For this review, take the finished solid that the model builds, in its own axes (mm). A direction names the side the tool comes from. Give positions to 0.01 mm unless a question says otherwise; leave off trailing zeros. Order: outer loops, then holes, each group sorted by start corner. A loop starts at its lowest first (then second) coordinate and runs counter-clockwise, first axis right, second up. Notation, with made-up numbers: (45.25, 40.25) - (54.25, 40.25) arc R23 ccw to (54.25, 67.25) - close; hole circle Ø5 at (0, -5.75). An arc over 180 degrees is marked (long way). Use a Markdown table: item, result. Add a question column.
1) We need section C-C on z = -87.5. Write out the cut boundary in (x, y).
2) Wall thickness on L1, parallel to Z at x = -18, y = 3.75; L2, parallel to X at y = 2.5, z = -98.5; L3, parallel to X at y = 3.25, z = -45.5: over which ranges is each line inside the solid? List them lowest first.
3) Clearance check with flat-ended pins moving along their axes: P1, Ø3.5, axis at x = -18.01, z = -37.86, coming from the +Y side; P2, Ø2, axis at y = 2.5, z = -77, coming from the +X side. State where each tip first meets the part, or that it passes through.
4) Mouldability with a two-part tool opening along Z and no side actions: class faces 4 (the face through (-37, 3, -102.633)), 5 (the face through (28.728, 3, -68)), 6 (the face through (-37, 3, -32.783)), 7 (the face through (-39, 6.35, -68)) as released by +Z, released by -Z, zero draft, split by the parting line, or undercut.
5) We need section A-A on y = 2.5. Give the number of separate pieces and of enclosed holes in the cut face, then the cut area to 3 significant figures.
6) Machinability: for faces 1 (the face through (33.35, 3.22, -90.36)), 2 (the face through (-105.395, 3, -68)), 3 (the face through (-57.8, 3.22, -36.23)), which of the approach directions +Z, -Z, +X, -X, +Y, -Y give a long, thin tool a straight path to every point of the face, cutting with its end or side? Answer none if there is none.
7) We need section B-B on z = -68. Write out the cut boundary in (x, y).
```python
from build123d import *

# Parameters (mm, degrees)
SKETCH1_W           = 67.061286962
SKETCH1_H           = 69.85
SKETCH1_R           = 1.27
BOSS_EXTRUDE1_DEPTH = 6.35
SKETCH2_W           = 20.976278342
SKETCH2_H           = 20.060000012
BOSS_EXTRUDE2_DEPTH = 12.7
BOSS_EXTRUDE3_DEPTH = 6.35
SKETCH4_W           = 170.998259203
SKETCH4_H           = 17.997071231
CUT_EXTRUDE1_DEPTH  = 70.85
SKETCH8_R           = 1.8415
CUT_EXTRUDE3_DEPTH  = 13.716


with BuildPart() as part:
    # Sketch1 → Boss-Extrude1 (new body)
    with BuildSketch(Plane(origin=(0, 0, 0), x_dir=(1, 0, 0), z_dir=(0, 1, 0))):
        with Locations((-4.803022, 67.707661351)):
            Rectangle(SKETCH1_W, SKETCH1_H)
        with Locations((3.381343157, 90.407661351)):
            Circle(SKETCH1_R, mode=Mode.SUBTRACT)
        with Locations((18.621343157, 90.407661351)):
            Circle(SKETCH1_R, mode=Mode.SUBTRACT)
        with Locations((3.381343157, 44.947661351)):
            Circle(SKETCH1_R, mode=Mode.SUBTRACT)
        with Locations((18.621343157, 44.947661351)):
            Circle(SKETCH1_R, mode=Mode.SUBTRACT)
    boss_extrude1 = extrude(amount=BOSS_EXTRUDE1_DEPTH)

    # Sketch2 → Boss-Extrude2 (add)
    with BuildSketch(Plane(origin=(0, 6.35, 0), x_dir=(1, 0, 0), z_dir=(0, 1, 0))):
        with Locations((18.23948231, 67.707661351)):
            Rectangle(SKETCH2_W, SKETCH2_H)
    boss_extrude2 = extrude(amount=BOSS_EXTRUDE2_DEPTH)

    # Sketch3 → Boss-Extrude3 (add)
    with BuildSketch(Plane(origin=(0, 6.35, 0), x_dir=(1, 0, 0), z_dir=(0, 1, 0))):
        Polygon((37.841343157, 102.632661351), (28.727621481, 77.737661357), (28.727621481, 102.632661351), align=None)
        Polygon((28.727621481, 57.677661345), (37.841343157, 32.782661351), (28.727621481, 32.782661351), align=None)
    boss_extrude3 = extrude(amount=-BOSS_EXTRUDE3_DEPTH)

    # Mirror2: Boss-Extrude1, Boss-Extrude2, Boss-Extrude3 across plane
    add(boss_extrude1.mirror(Plane(origin=(-38.333665481, 6.35, -32.782661351), x_dir=(0, 0, 1), z_dir=(1, 0, 0))))
    add(boss_extrude2.mirror(Plane(origin=(-38.333665481, 6.35, -32.782661351), x_dir=(0, 0, 1), z_dir=(1, 0, 0))))
    add(boss_extrude3.mirror(Plane(origin=(-38.333665481, 6.35, -32.782661351), x_dir=(0, 0, 1), z_dir=(1, 0, 0))))

    # Sketch4 → Cut-Extrude1 (cut, through all)
    with BuildSketch(Plane.XY.offset(-32.782661351)):
        with Locations((-47.657786445, 15.348535616)):
            Rectangle(SKETCH4_W, SKETCH4_H)
    extrude(amount=-CUT_EXTRUDE1_DEPTH, mode=Mode.SUBTRACT)

    # Sketch8 → Cut-Extrude3 (cut)
    with BuildSketch(Plane(origin=(0, 6.35, 0), x_dir=(1, 0, 0), z_dir=(0, 1, 0))):
        with Locations((-58.653665481, 97.552661351)):
            Circle(SKETCH8_R)
        with Locations((-18.013665481, 97.552661351)):
            Circle(SKETCH8_R)
        with Locations((-18.013665481, 37.862661351)):
            Circle(SKETCH8_R)
        with Locations((-58.653665481, 37.862661351)):
            Circle(SKETCH8_R)
    extrude(amount=-CUT_EXTRUDE3_DEPTH, mode=Mode.SUBTRACT)


solid = part.part
```
Checked values:
| question | item | result |
|---|---|---|
| 1 | outline | (-108.97, 0) - (32.3, 0) - (32.3, 6.35) - (-108.97, 6.35) - close |
| 2 | L1 | -102.63 to -99.39, -95.71 to -39.7, -36.02 to -32.78 |
| 2 | L2 | -113 to -60.23, -57.07 to -19.59, -16.43 to 36.33 |
| 2 | L3 | -109.85 to -96.43, -94.15 to -81.19, -78.91 to 2.24, 4.52 to 17.48, 19.76 to 33.19 |
| 3 | P1 | through |
| 3 | P2 | x = 28.82 |
| 4 | face 4 | released by -Z |
| 4 | face 5 | undercut |
| 4 | face 6 | released by +Z |
| 4 | face 7 | zero draft |
| 5 | separate pieces | 1 |
| 5 | enclosed holes | 12 |
| 5 | area | 9,740 mm² |
| 6 | face 1 | +X, +Y, -Y |
| 6 | face 2 | -X, +Y, -Y |
| 6 | face 3 | +Y, -Y |
| 7 | outline | (-105.39, 0) - (28.73, 0) - (28.73, 6.35) - (-105.39, 6.35) - close |
